Could you check a few things on this model? Use its own coordinates, in mm. A direction names the side the tool comes from. Give positions to 0.01 mm unless a question says otherwise; leave off trailing zeros. Order: outer loops, then holes, each group sorted by start corner. A loop starts at its lowest first (then second) coordinate and runs counter-clockwise, first axis right, second up. Notation, with made-up numbers: M 62.5,72.5 L 94.5,72.5 A15 cw 94.5,90.5 Z; hole C 25,24 d1. An arc over 180 degrees is marked long. Answer in a Markdown table with one row per item. Add a question column.
Autodesk Inventor part; units mm, degrees
ref_plane "YZ Plane" through (0, 0, 0) normal (1, 0, 0) x (0, 1, 0)
ref_plane "XZ Plane" through (0, 0, 0) normal (0, 1, 0) x (-1, 0, 0)
ref_plane "XY Plane" through (0, 0, 0) normal (0, 0, 1) x (1, 0, 0)
sketch "Эскиз1" plane through (0, 0, 0) normal (0, 1, 0) x (-1, 0, 0)
  line L0 (43.5, 4) -> (43.5, -6)
  line L1 (43.5, -6) -> (39.5, -6)
  line L2 (39.5, -6) -> (39.5, -20)
  line L3 (39.5, -20) -> (27.5, -20)
  line L4 (27.5, -20) -> (27.5, -16)
  line L5 (27.5, -16) -> (7.5, -16)
  line L6 (7.5, -16) -> (7.5, -20)
  line L7 (7.5, -20) -> (0, -20)
  line L8 (0, -20) -> (0, 0)
  line L9 (-43.5, 4) -> (-43.5, -6)
  line L10 (-43.5, -6) -> (-39.5, -6)
  line L11 (-39.5, -6) -> (-39.5, -20)
  line L12 (-39.5, -20) -> (-27.5, -20)
  line L13 (-27.5, -20) -> (-27.5, -16)
  line L14 (-27.5, -16) -> (-7.5, -16)
  line L15 (-7.5, -16) -> (-7.5, -20)
  line L16 (-7.5, -20) -> (0, -20)
  line L17 (43.5, 4) -> (20, 4)
  line L18 (20, 4) -> (20, 0)
  line L19 (20, 0) -> (0, 0)
  line L20 (-43.5, 4) -> (-20, 4)
  line L21 (-20, 4) -> (-20, 0)
  line L22 (-20, 0) -> (0, 0)
  dimension "d0" = 12
  dimension "d1" = 20
  dimension "d2" = 15
  dimension "d3" = 4
  dimension "d4" = 14
  dimension "d5" = 10
  dimension "d8" = 40
extrude "Выдавливание1" add sketch "Эскиз1" along normal blind 4
properties part number "batN" material "Дерево (береза)"
1. If I drill on line 1 along X through (y, z) = (0.5, -16.75); line 2 along X through (y, z) = (0.8, 0.75); line 3 along Z through (x, y) = (-14.5, 1), over which ranges is the centre line in solid material (lowest first)? Write a range as [from, to].
2. Suppose I cut it at C-C on x = 2. List the corners of the cut face in (y, z) for me, plus the area to 3 significant figures.
3. Suppose I cut it at A-A on z = 2.25. List the corners of the cut face in (x, y) for me.
4. For faces 4 (the flat face through (18, 2, -16)), 5 (the flat face through (42, 2, -6)), 6 (the flat face through (0, 2, 0)), which set-ups out of +Z, -Z, +X, -X, +Y, -Y let a thin tool reach every point of the face, with its end or its side?
5. Suppose I cut it at B-B on y = 1.6. List the corners of the cut face in (x, z) for me.
6. Suppose I cut it at D-D on z = -13. List the corners of the cut face in (x, y) for me, plus the area to 3 significant figures.
7. Will these pins go through, and if not, where does the flat tip stop? P1, Ø2, axis at y = 1.5, z = -15.5, coming from the -X side; P2, Ø2, axis at y = 2.5, z = -17, coming from the +X side; P3, Ø1.2, axis at x = 42, y = 2, coming from the -Z side.
8. Thinking about a two-plate mould opening in X: for faces 1 (the flat face through (-43.5, 2, -1)), 2 (the flat face through (-32, 2, 4)), 3 (the flat face through (-18, 2, -16)), which applies, pulls with the +X half, pulls with the -X half, needs draft (parallel to the pull), parting line crosses it, or undercut?
Findings below:
| question | item | result |
|---|---|---|
| 1 | line 1 | [-39.5, -27.5], [-7.5, 7.5], [27.5, 39.5] |
| 1 | line 2 | [-43.5, -20], [20, 43.5] |
| 1 | line 3 | [-16, 0] |
| 2 | outline | M 0,-20 L 4,-20 L 4,0 L 0,0 Z |
| 2 | area | 80.0 mm2 |
| 3 | outline | M -43.5,0 L -20,0 L -20,4 L -43.5,4 Z; M 20,0 L 43.5,0 L 43.5,4 L 20,4 Z |
| 4 | face 4 | -Z, +Y, -Y |
| 4 | face 5 | -Z, +X, +Y, -Y |
| 4 | face 6 | +Z, +Y, -Y |
| 5 | outline | M -43.5,-6 L -39.5,-6 L -39.5,-20 L -27.5,-20 L -27.5,-16 L -7.5,-16 L -7.5,-20 L 7.5,-20 L 7.5,-16 L 27.5,-16 L 27.5,-20 L 39.5,-20 L 39.5,-6 L 43.5,-6 L 43.5,4 L 20,4 L 20,0 L -20,0 L -20,4 L -43.5,4 Z |
| 6 | outline | M -39.5,0 L 39.5,0 L 39.5,4 L -39.5,4 Z |
| 6 | area | 316 mm2 |
| 7 | P1 | x = -39.5 |
| 7 | P2 | x = 39.5 |
| 7 | P3 | z = -6 |
| 8 | face 1 | pulls with the -X half |
| 8 | face 2 | needs draft |
| 8 | face 3 | undercut |
